Part model, mm, in its own coordinate system. Face numbers are marked on the shaded views. A direction names the side the tool comes from. Give positions to 0.01 mm unless a question says otherwise; leave off trailing zeros. Write each loop counter-clockwise with the first axis right and the second up, starting at its lowest first coordinate (ties: lowest second). Pieces come first, ordered by that corner, then holes. Notation, with made-up numbers: M 75,89 L 106,89 A18 ccw 106,122 Z; hole C 45,-10 d4. An arc over 180 degrees is marked long. Write item = value, one per line. Start each with the question number.
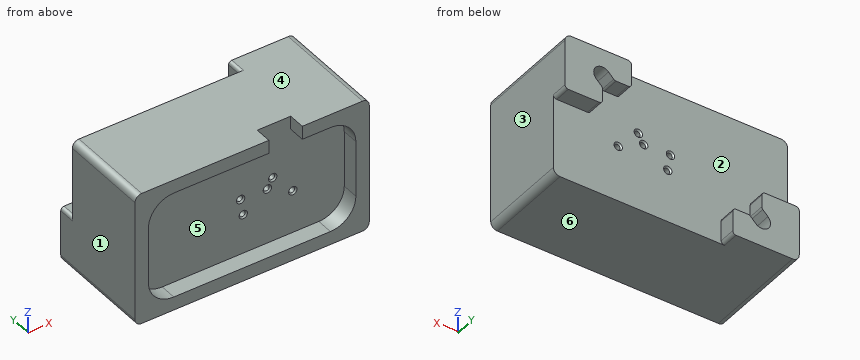
from build123d import *

# Parameters (mm, degrees)
SKETCH1_W                            = 44.45
SKETCH1_H                            = 25.4
BOSS_EXTRUDE1_DEPTH                  = 17.145
BOSS_EXTRUDE2_DEPTH                  = 3.175
CUT_EXTRUDE1_DEPTH                   = 3.175
F_57_0_043_DIAMETER_HOLE1_AT_2_COUNT = 2
F_57_0_043_DIAMETER_HOLE1_AT_2_PITCH = 5.663972193
F_57_0_043_DIAMETER_HOLE1_AT_3_COUNT = 2
F_57_0_043_DIAMETER_HOLE1_AT_3_PITCH = 5.39563203
F_57_0_043_DIAMETER_HOLE1_AT_4_COUNT = 2
F_57_0_043_DIAMETER_HOLE1_AT_4_PITCH = 10.226457647
F_57_0_043_DIAMETER_HOLE1_AT_5_COUNT = 2
F_57_0_043_DIAMETER_HOLE1_AT_5_PITCH = 9.419428274
FILLET1_R                            = 0.635
FILLET2_R                            = 1.27
FILLET3_R                            = 4.826


with BuildPart() as part:
    # Sketch1 → Boss-Extrude1 (new body)
    with BuildSketch(Plane(origin=(0, 0, 0), x_dir=(1, 0, 0), z_dir=(0, 1, 0))):
        Rectangle(SKETCH1_W, SKETCH1_H)
    extrude(amount=BOSS_EXTRUDE1_DEPTH)

    # Sketch2 → Boss-Extrude2 (add)
    with BuildSketch(Plane(origin=(0, 17.145, 0), x_dir=(1, 0, 0), z_dir=(0, 1, 0))):
        with BuildLine():
            Line((-22.225, 12.7), (-9.615133409, 12.7))
            Line((-9.615133409, 12.7), (-9.615133409, 7.625))
            Line((-9.615133409, 7.625), (-12.790133409, 7.625))
            Line((-12.790133409, 7.625), (-13.957566704, 8.792433296))
            ThreePointArc((-13.957566704, 8.792433296), (-16.292433296, 8.792433296), (-16.292433296, 6.457566704))
            Line((-16.292433296, 6.457566704), (-15.125, 5.290133409))
            Line((-15.125, 5.290133409), (-15.125, 2.115133409))
            Line((-15.125, 2.115133409), (-22.225, 2.115133409))
            Line((-22.225, 2.115133409), (-22.225, 12.7))
        make_face()
        with BuildLine():
            Line((22.225, -12.7), (22.225, -2.115133409))
            Line((22.225, -2.115133409), (15.125, -2.115133409))
            Line((15.125, -2.115133409), (15.125, -5.290133409))
            Line((15.125, -5.290133409), (16.292433296, -6.457566704))
            ThreePointArc((16.292433296, -6.457566704), (16.292433296, -8.792433296), (13.957566704, -8.792433296))
            Line((13.957566704, -8.792433296), (12.790133409, -7.625))
            Line((12.790133409, -7.625), (9.615133409, -7.625))
            Line((9.615133409, -7.625), (9.615133409, -12.7))
            Line((9.615133409, -12.7), (22.225, -12.7))
        make_face()
    extrude(amount=BOSS_EXTRUDE2_DEPTH)

    # Sketch6 → Cut-Extrude1 (cut)
    with BuildSketch(Plane.XZ):
        Polygon((3.175, 10.16), (3.175, 12.7), (9.525, 12.7), (9.525, 10.16), (19.685, 10.16), (19.685, -10.16), (-19.685, -10.16), (-19.685, 10.16), align=None)
    extrude(amount=-CUT_EXTRUDE1_DEPTH, mode=Mode.SUBTRACT)

    # Sketch4 → #57 (0.043) Diameter Hole1 (revolve, cut)
    with BuildSketch(Plane(origin=(9.92, 17.145, -2.025), x_dir=(0, 0, 1), z_dir=(1, 0, 0))):
        Polygon((0, 0), (0, 13.97), (0.79375, 13.97), (0.5461, 13.685111264), (0.5461, 0.284888736), (0.79375, 0), align=None)
    f_57_0_043_diameter_hole1 = revolve(axis=Axis((9.92, 23.495, -2.025), (0, -1, 0)), mode=Mode.SUBTRACT)

    # #57 (0.043) Diameter Hole1 at 2: #57 (0.043) Diameter Hole1 ×2
    with Locations(*[Vector(-0.6726727939963121, 0, 0.7399400733959441) * (i * F_57_0_043_DIAMETER_HOLE1_AT_2_PITCH) for i in range(1, F_57_0_043_DIAMETER_HOLE1_AT_2_COUNT)]):
        add(f_57_0_043_diameter_hole1, mode=Mode.SUBTRACT)

    # #57 (0.043) Diameter Hole1 at 3: #57 (0.043) Diameter Hole1 ×2
    with Locations(*[Vector(-0.894427190999916, 0, 0.447213595499958) * (i * F_57_0_043_DIAMETER_HOLE1_AT_3_PITCH) for i in range(1, F_57_0_043_DIAMETER_HOLE1_AT_3_COUNT)]):
        add(f_57_0_043_diameter_hole1, mode=Mode.SUBTRACT)

    # #57 (0.043) Diameter Hole1 at 4: #57 (0.043) Diameter Hole1 ×2
    with Locations(*[Vector(-0.968663866044045, 0, 0.24837535026770383) * (i * F_57_0_043_DIAMETER_HOLE1_AT_4_PITCH) for i in range(1, F_57_0_043_DIAMETER_HOLE1_AT_4_COUNT)]):
        add(f_57_0_043_diameter_hole1, mode=Mode.SUBTRACT)

    # #57 (0.043) Diameter Hole1 at 5: #57 (0.043) Diameter Hole1 ×2
    with Locations(*[Vector(-0.9977250982863921, 0, -0.06741385799232386) * (i * F_57_0_043_DIAMETER_HOLE1_AT_5_PITCH) for i in range(1, F_57_0_043_DIAMETER_HOLE1_AT_5_COUNT)]):
        add(f_57_0_043_diameter_hole1, mode=Mode.SUBTRACT)

    # Fillet1
    fillet1_edges = [part.edges().sort_by_distance(p)[0] for p in [
        (9.615133409, 18.7325, 12.7),
        (22.225, 18.7325, 2.115133409),
        (9.615133409, 18.7325, 7.625),
        (12.790133409, 18.7325, 7.625),
        (15.125, 18.7325, 5.290133409),
        (15.125, 18.7325, 2.115133409),
        (-9.615133409, 18.7325, -12.7),
        (-9.615133409, 18.7325, -7.625),
        (-12.790133409, 18.7325, -7.625),
        (-15.125, 18.7325, -5.290133409),
        (-15.125, 18.7325, -2.115133409),
        (-22.225, 18.7325, -2.115133409),
    ]]
    fillet(fillet1_edges, radius=FILLET1_R)

    # Fillet2
    fillet2_edges = [part.edges().sort_by_distance(p)[0] for p in [
        (22.225, 8.5725, -12.7),
        (22.225, 10.16, 12.7),
        (-22.225, 8.5725, 12.7),
        (-22.225, 10.16, -12.7),
    ]]
    fillet(fillet2_edges, radius=FILLET2_R)

    # Fillet3
    fillet3_edges = [part.edges().sort_by_distance(p)[0] for p in [
        (-19.685, 1.5875, 10.16),
        (19.685, 1.5875, 10.16),
        (19.685, 1.5875, -10.16),
        (-19.685, 1.5875, -10.16),
    ]]
    fillet(fillet3_edges, radius=FILLET3_R)


solid = part.part
Q1. Probe line 1 along X through (y, z) = (2.75, -0.5) (3 decimals); line 2 along Z through (x, y) = (9.92, 6.5); line 3 along Z through (x, y) = (-1, 2.5). List the from-to ranges inside material, lowest first.
Q2. Drop flat-ended pins along their axis: P1, Ø1.5, axis at x = -3.5, z = -5.5, coming from the +Y side (3 decimals); P2, Ø10, axis at x = 9, z = 8.5, coming from the -Y side; P3, Ø1.4, axis at x = 9.92, z = -2.025, coming from the +Y side; P4, Ø1.1, axis at x = -11.5, y = 19.5, coming from the +Z side (3 decimals). Give the stop position or say it passes through.
Q3. Tool access for the marked faces 1 and 2: list every direction of +Z, -Z, +X, -X, +Y, -Y with a clear straight run to the whole face (end or side of a thin tool).
Q4. Slice it at A-A (y = 2.5). Give the cut face in (x, z) (3 decimals).
Q5. Slice it at B-B (x = 8). Give the cut face in (y, z) (3 decimals).
Q6. Slice it at C-C (x = 19). Give the cut face in (y, z) (3 decimals), and give its area (3 significant figures).
Q7. Two-plate mould, pull along Z, no slides. Class the marked faces 3, 4, 5 and 6: +Z half, -Z half, draft (parallel to the pull), parting line (faces both ways), or undercut.
Working result:
q1.line_1 = -22.225 to -19.685, 19.685 to 22.225
q1.line_2 = -12.7 to -2.57, -1.48 to 12.7
q1.line_3 = -12.7 to -10.16, 10.16 to 12.7
q2.P1 = 17.145
q2.P2 = 0
q2.P3 = 17.04
q2.P4 = -7.625
q3.face_1 = +Z, -Z, -X, +Y, -Y
q3.face_2 = +Y
q4.outline = M -22.225,-11.43 A1.27 ccw -20.955,-12.7 L 20.955,-12.7 A1.27 ccw 22.225,-11.43 L 22.225,11.43 A1.27 ccw 20.955,12.7 L 9.525,12.7 L 9.525,10.16 L 14.859,10.16 A4.826 cw 19.685,5.334 L 19.685,-5.334 A4.826 cw 14.859,-10.16 L -14.859,-10.16 A4.826 cw -19.685,-5.334 L -19.685,5.334 A4.826 cw -14.859,10.16 L 3.175,10.16 L 3.175,12.7 L -20.955,12.7 A1.27 ccw -22.225,11.43 Z
q5.outline = M 0,-12.7 L 17.145,-12.7 L 17.145,12.7 L 3.175,12.7 L 3.175,-10.16 L 0,-10.16 Z
q6.outline = M 0,-12.7 L 17.145,-12.7 L 17.145,2.115 L 20.32,2.115 L 20.32,12.7 L 0,12.7 L 0,7.812 L 3.175,7.812 L 3.175,-7.812 L 0,-7.812 Z
q6.area = 419 mm2
q7.face_3 = draft
q7.face_4 = +Z half
q7.face_5 = undercut
q7.face_6 = -Z half
